from build123d import *

# Parameters (mm, degrees)
SKETCH2_W           = 17
SKETCH2_H           = 26
BOSS_EXTRUDE1_DEPTH = 1
SKETCH3_R           = 0.825554505
SKETCH3_R_2         = 0.799067601
SKETCH3_R_3         = 0.4
SKETCH3_R_4         = 0.016836885
SKETCH3_W           = 3.624022482
SKETCH3_H           = 3.358967559
SKETCH3_W_2         = 2.916998144
SKETCH3_H_2         = 3.005392027
SKETCH3_W_3         = 3.9335278
SKETCH3_H_3         = 3.447361443
SKETCH3_W_4         = 0.928135773
SKETCH3_H_4         = 0.662954124
SKETCH3_W_5         = 0.883938831
SKETCH3_H_5         = 0.972332715
SKETCH3_W_6         = 2.524073743
SKETCH3_H_6         = 3.291762325
SKETCH3_H_7         = 0.574560241
SKETCH3_H_8         = 0.82518615
SKETCH3_H_9         = 0.486166357
SKETCH3_W_7         = 2.696013436
SKETCH3_H_10        = 1.635286838
SKETCH3_W_8         = 2.033059313
SKETCH3_H_11        = 0.972332714
SKETCH3_H_12        = 0.707151065
SKETCH3_W_9         = 1.676172691
SKETCH3_H_13        = 2.519225669
SKETCH3_W_10        = 0.670281766
SKETCH3_H_14        = 1.583920148
BOSS_EXTRUDE2_DEPTH = 1
SKETCH4_R           = 1.59
SKETCH4_R_2         = 0.42
CUT_EXTRUDE1_DEPTH  = 3
SKETCH5_W           = 2.209847079
SKETCH5_H           = 2.696013435
BOSS_EXTRUDE3_DEPTH = 2


with BuildPart() as part:
    # Sketch2 → Boss-Extrude1 (new body)
    with BuildSketch(Plane(origin=(0, 0, 0), x_dir=(1, 0, 0), z_dir=(0, 1, 0))):
        Rectangle(SKETCH2_W, SKETCH2_H)
    extrude(amount=BOSS_EXTRUDE1_DEPTH)

    # Sketch3 → Boss-Extrude2 (add)
    with BuildSketch(Plane(origin=(0, 1, 0), x_dir=(1, 0, 0), z_dir=(0, 1, 0))):
        with Locations((-6, -10.5)):
            Circle(SKETCH3_R)
        with Locations((-6, 10.5)):
            Circle(SKETCH3_R_2)
        with Locations((7.26674642, 11.385525432)):
            Circle(SKETCH3_R_3)
        with Locations((7.26674642, 11.385525432)):
            Circle(SKETCH3_R_4, mode=Mode.SUBTRACT)
        with Locations((2.519162306, 10.342084328)):
            Rectangle(SKETCH3_W, SKETCH3_H)
        with Locations((3.800810248, 6.010784054)):
            Rectangle(SKETCH3_W_2, SKETCH3_H_2)
        with Locations((-2.232072277, 6.541147353)):
            Rectangle(SKETCH3_W_3, SKETCH3_H_3)
        with Locations((-4.132540764, 3.292672147)):
            Rectangle(SKETCH3_W_4, SKETCH3_H_4)
        with Locations((-1.237641092, 3.137982852)):
            Rectangle(SKETCH3_W_5, SKETCH3_H_5)
        with Locations((0.024395781, -0.364169856)):
            Rectangle(SKETCH3_W_6, SKETCH3_H_6)
        with Locations((-4.132540764, 0.994431186)):
            Rectangle(SKETCH3_W_4, SKETCH3_H_7)
        with Locations((-4.132540764, -0.412593075)):
            Rectangle(SKETCH3_W_4, SKETCH3_H_8)
        with Locations((-4.132540764, -2.54132414)):
            Rectangle(SKETCH3_W_4, SKETCH3_H_9)
        with Locations((0.110365627, -4.972155927)):
            Rectangle(SKETCH3_W_7, SKETCH3_H_10)
        with Locations((4.242779664, 1.767877663)):
            Rectangle(SKETCH3_W_8, SKETCH3_H_11)
        with Locations((4.242779664, -0.883938832)):
            Rectangle(SKETCH3_W_8, SKETCH3_H_12)
        with Locations((3.386837508, -9.126668435)):
            Rectangle(SKETCH3_W_9, SKETCH3_H_13)
        with Locations((0.335140883, -9.498757564)):
            Rectangle(SKETCH3_W_10, SKETCH3_H_14)
    extrude(amount=BOSS_EXTRUDE2_DEPTH)

    # Sketch4 → Cut-Extrude1 (cut, through all)
    with BuildSketch(Plane(origin=(0, 2, 0), x_dir=(1, 0, 0), z_dir=(0, 1, 0))):
        with Locations((-6, 10.5)):
            Circle(SKETCH4_R)
        with Locations((-6, -10.5)):
            Circle(SKETCH4_R)
        with Locations((7.26674642, 11.385525432)):
            Circle(SKETCH4_R_2)
        with Locations((7.26674642, 8.885525432)):
            Circle(SKETCH4_R_2)
        with Locations((7.26674642, 6.385525432)):
            Circle(SKETCH4_R_2)
        with Locations((7.26674642, 3.885525432)):
            Circle(SKETCH4_R_2)
        with Locations((7.26674642, 1.385525432)):
            Circle(SKETCH4_R_2)
        with Locations((7.26674642, -1.114474568)):
            Circle(SKETCH4_R_2)
        with Locations((7.26674642, -3.614474568)):
            Circle(SKETCH4_R_2)
        with Locations((7.26674642, -6.114474568)):
            Circle(SKETCH4_R_2)
        with Locations((7.26674642, -8.614474568)):
            Circle(SKETCH4_R_2)
        with Locations((7.26674642, -11.114474568)):
            Circle(SKETCH4_R_2)
    extrude(amount=-CUT_EXTRUDE1_DEPTH, mode=Mode.SUBTRACT)

    # Sketch5 → Boss-Extrude3 (add)
    with BuildSketch(Plane(origin=(0, 1, 0), x_dir=(1, 0, 0), z_dir=(0, 1, 0))):
        with Locations((4.19870945, -5.104746752)):
            Rectangle(SKETCH5_W, SKETCH5_H)
    extrude(amount=BOSS_EXTRUDE3_DEPTH)


solid = part.part
The model under review builds one solid part; all positions refer to its coordinate system, in mm. A direction names the side the tool comes from. Round coordinates to 2 decimals unless told otherwise and drop trailing zeros. Loops run counter-clockwise (first coordinate to the right, second up) from the corner with the lowest first, then second, coordinate; pieces in that order, holes last. Notation, with made-up numbers: M 72.5,-39 L 83.5,-39 A36 ccw 83.5,-1 Z; hole C -39.75,89 d8. An arc over 180 degrees is marked long. Answer as CSV lines item,"result". Start each with the question number.
Item 1: Mouldability with a two-part tool opening along X and no side actions: class faces 4 (the face through (-0.796, 1.5, -3.1)), 5 (the face through (4, 2, 6.453)), 6 (the face through (6.96, 0.51, 3.33)), 7 (the face through (7.176, 0.507, 6.524)) as released by +X, released by -X, zero draft, split by the parting line, or undercut.
Item 2: For faces 1 (the face through (0.67, 1.5, 9.5)), 2 (the face through (3.4, 1.5, 7.867)), 3 (the face through (-1.238, 1.5, 5)), list the 3-axis set-ups (+Z, -Z, +X, -X, +Y, -Y) from which the entire face can be reached by the end or side of a thin tool; tool diameter is ignored.
Item 3: Consider section C-C (x = -2.25). Write out the cut boundary in (y, z), then the cut area to 3 significant figures.
Item 4: Consider section A-A (z = -10.5). Write out the cut boundary in (x, y), then the cut area to 3 significant figures.
Item 5: Wall thickness on line 1 (Z direction, x = -6, y = 0.3); line 2 (X direction, y = 0.2, z = 10.5); line 3 (Z direction, x = 3.75, y = 1.5): over which ranges is each line inside the solid? List them lowest first. Write a range as [from, to].
Item 6: Consider section D-D (y = 1.5). State how many separate pieces and enclosed holes the cut face has, then the cut area to 3 significant figures.
Item 7: Insertion check: P1, Ø0.8, axis at y = 1.5, z = 9.5, coming from the +X side; P2, Ø0.7, axis at x = -1, y = 1.5, coming from the +Z side; P3, Ø0.6, axis at y = 2, z = 4.5, coming from the -X side. Each pin has a flat end and moves straight along its axis. Give the tip position at first contact, or say it passes through.
Item 8: Consider section B-B (x = -6). Write out the cut boundary in (y, z).
Answer:
1,face 4,"released by +X"
1,face 5,"zero draft"
1,face 6,"undercut"
1,face 7,"undercut"
2,face 1,"+Z, +Y"
2,face 2,"+X, -X, +Y"
2,face 3,"+Z, -X, +Y"
3,outline,"M 0,-13 L 1,-13 L 1,-8.26 L 2,-8.26 L 2,-4.82 L 1,-4.82 L 1,13 L 0,13 Z"
3,area,"29.4 mm^2"
4,outline,"M -8.5,0 L -7.59,0 L -7.59,1 L -8.5,1 Z; M -4.41,0 L 8.5,0 L 8.5,1 L 4.33,1 L 4.33,2 L 0.71,2 L 0.71,1 L -4.41,1 Z"
4,area,"17.4 mm^2"
5,line 1,"z = [-13, -12.09], [-8.91, 8.91], [12.09, 13]"
5,line 2,"x = [-8.5, -7.59], [-4.41, 8.5]"
5,line 3,"z = [-12.02, -8.66], [-7.51, -4.51], [-2.25, -1.28], [0.53, 1.24], [3.76, 6.45], [7.87, 10.39]"
6,separate pieces,"15"
6,enclosed holes,"0"
6,area,"65.1 mm^2"
7,P1,"stops at x = 4.22"
7,P2,"stops at z = 5.79"
7,P3,"stops at x = -1.24"
8,outline,"M 0,-13 L 1,-13 L 1,-12.09 L 0,-12.09 Z; M 0,-8.91 L 1,-8.91 L 1,8.91 L 0,8.91 Z; M 0,12.09 L 1,12.09 L 1,13 L 0,13 Z"
